```python
from build123d import *

# Parameters (mm, degrees)
SKETCH004_R  = 7.93
PAD_DEPTH    = 16
SKETCH005_R  = 7.5
PAD001_DEPTH = 6
SKETCH006_R  = 7.4
PAD002_DEPTH = 85
SKETCH007_R  = 7.5
PAD003_DEPTH = 8
SKETCH008_R  = 7.4
PAD004_DEPTH = 20


with BuildPart() as part:
    # Sketch004 → Pad (new body)
    with BuildSketch(Plane.XY):
        Circle(SKETCH004_R)
    extrude(amount=PAD_DEPTH)

    # Sketch005 → Pad001 (new body)
    with BuildSketch(Plane.XY.offset(16)):
        Circle(SKETCH005_R)
    extrude(amount=PAD001_DEPTH)

    # Sketch006 → Pad002 (new body)
    with BuildSketch(Plane.XY.offset(22)):
        Circle(SKETCH006_R)
    extrude(amount=PAD002_DEPTH)

    # Sketch007 → Pad003 (new body)
    with BuildSketch(Plane.XY.offset(107)):
        Circle(SKETCH007_R)
    extrude(amount=PAD003_DEPTH)

    # Sketch008 → Pad004 (new body)
    with BuildSketch(Plane.XY.offset(115)):
        Circle(SKETCH008_R)
    extrude(amount=PAD004_DEPTH)


solid = part.part
```
Check sheet for the modelled part. Datum: model origin and axes. Units: mm. A direction names the side the tool comes from. Round coordinates to 2 decimals unless told otherwise and drop trailing zeros. Loops run counter-clockwise (first coordinate to the right, second up) from the corner with the lowest first, then second, coordinate; pieces in that order, holes last. Notation, with made-up numbers: (-39.5, 47) - (12.5, 47) arc R9 ccw to (12.5, 56) - close; hole circle Ø3 at (22, 40). An arc over 180 degrees is marked (long way). Write item = value, one per line. Start each with the question number.
Q1. Section check C-C (z = 80). Record the boundary of the cut face in (x, y), plus the area to 3 significant figures.
Q2. Release check for a two-part mould opening along Z. For faces 1 (the face through (-7.493, 0.33, 18.958)), 2 (the face through (0, 0, 135)), 3 (the face through (0, 0, 0)), 4 (the face through (-1.604, -7.224, 63.905)) record: pulls with the +Z half, pulls with the -Z half, needs draft (parallel to the pull), parting line crosses it, or undercut.
Q3. Section check A-A (y = 0). Record the boundary of the cut face in (x, z), plus the area to 3 significant figures.
Q4. Thickness scan on L1, parallel to Y at x = -0.5, z = 79.5; L2, parallel to Z at x = 7.25, y = -2.25; L3, parallel to Y at x = 4.5, z = 54. Record the ranges inside material, lowest first.
Q5. Depth check by flat-ended pin: P1, Ø5, axis at x = 2.5, z = 44.5, coming from the -Y side; P2, Ø8, axis at y = -4, z = 121, coming from the -X side; P3, Ø1, axis at y = -3.5, z = 39.5, coming from the +X side; P4, Ø3, axis at x = 6, y = 2, coming from the -Z side. Enter the tip coordinate at first touch or a pass-through.
Q6. Access from +Z, -Z, +X, -X, +Y, -Y to the whole of each face (thin tool, end or side, straight path). Record for faces 5 (the face through (-6.29, -4.83, 7.89)), 6 (the face through (-1.604, -7.224, 124.86)).
Derived:
q1.outline = circle Ø14.8 at (0, 0)
q1.area = 172 mm^2
q2.face_1 = needs draft
q2.face_2 = pulls with the +Z half
q2.face_3 = pulls with the -Z half
q2.face_4 = undercut
q3.outline = (-7.93, 0) - (7.93, 0) - (7.93, 16) - (7.5, 16) - (7.5, 22) - (7.4, 22) - (7.4, 107) - (7.5, 107) - (7.5, 115) - (7.4, 115) - (7.4, 135) - (-7.4, 135) - (-7.4, 115) - (-7.5, 115) - (-7.5, 107) - (-7.4, 107) - (-7.4, 22) - (-7.5, 22) - (-7.5, 16) - (-7.93, 16) - close
q3.area = 2,020 mm^2
q4.L1 = -7.38 to 7.38
q4.L2 = 0 to 16
q4.L3 = -5.87 to 5.87
q5.P1 = -7.4
q5.P2 = -7.4
q5.P3 = 6.76
q5.P4 = 0
q6.face_5 = +Z, -Z
q6.face_6 = +Z
